Autodesk Inventor part; units mm, degrees
ref_plane "YZ Plane" through (0, 0, 0) normal (1, 0, 0) x (0, 1, 0)
ref_plane "XZ Plane" through (0, 0, 0) normal (0, 1, 0) x (-1, 0, 0)
ref_plane "XY Plane" through (0, 0, 0) normal (0, 0, 1) x (1, 0, 0)
sketch "草圖1" plane through (0, 0, 0) normal (1, 0, 0) x (0, 1, 0)
  line L0 (75, 0) -> (-75, 0)
  line L1 (-75, 0) -> (-75, -300)
  line L2 (-75, -300) -> (75, -300)
  line L3 (75, -300) -> (75, 0)
  circle A0 centre (0, -100) radius 15
  circle A1 centre (0, -150) radius 15
  circle A2 centre (0, -225) radius 30
  line L4 (75, -300) -> (-75, -300)
  line L5 (-75, -300) -> (-75, -725)
  line L6 (-75, -725) -> (75, -725)
  line L7 (75, -725) -> (75, -300)
  point P0 (0, 0)
  point P1 (0, 0)
  dimension "d0" = 150
  dimension "d1" = 300
  dimension "d2" = 200
  dimension "d3" = 50
  dimension "d4" = 75
  dimension "d5" = 60
  dimension "d6" = 30
  dimension "d7" = 500
extrude "擠出1" add sketch "草圖1" along normal mid plane 75
full round fillet "圓角1" first side at (-12.5, -75, -241.6667) centre faces at (12.5, -25, -725) second side at (-12.5, 75, -483.3333)
sketch "草圖2" plane through (37.5, 0, 0) normal (1, 0, 0) x (0, 0, -1)
  arc A0 (650, -75) -> (650, 75) centre (650, 0) ccw
  line L0 (650, 75) -> (0, 75)
  line L1 (0, 75) -> (0, -75)
  line L2 (0, -75) -> (650, -75)
  circle A1 centre (225, 0) radius 30
  circle A2 centre (150, 0) radius 15
  circle A3 centre (100, 0) radius 15
  circle A4 centre (650, 0) radius 200
  point P0 (0, 0)
  dimension "d10" = 400
extrude "擠出2" add sketch "草圖2" along normal blind 30 contours L2 A4 L0 A0 | A0 L0 A4 L2
fillet "圓角2" radius 75 2 edges at (0, 75, 0) (0, -75, 0)
properties part number "震動臂"
Input: part model. Units: mm. Frame: model coordinates. A direction names the side the tool comes from. Coordinates: 2 decimals unless noted, no trailing zeros. Loops run counter-clockwise (first coordinate to the right, second up) from the corner with the lowest first, then second, coordinate; pieces in that order, holes last.
Q1. Material intervals for line 1 (Z direction, x = 4, y = 0); line 2 (X direction, y = 150.5, z = -671.5); line 3 (Y direction, x = 21.5, z = -365.5), sorted ascending.
Q2. Cut plane D-D (y = -153). Output: boundary loops of the cut face in (x, z), then the cut area to 3 significant figures.
Q3. Draft query along Z for faces 5 (the face through (-0.52, 53.61, -702.45)), 6 (the face through (52.29, -8.794, -450.193)), 7 (the face through (-0.525, -3.252, -85.357)). Return one class per face: +Z half, -Z half, draft (parallel to the pull), parting line (faces both ways), or undercut.
Q4. Set-up query: faces 1 (the face through (37.5, 3, -740)), 2 (the face through (-1, -75, -358)), 3 (the face through (-1, 75, -367)), 4 (the face through (-0.52, -52.45, -703.61)). Return all of +Z, -Z, +X, -X, +Y, -Y with unobstructed straight access to the full face (end or side cutting, diameter ignored); none if empty.
Q5. Contact query for flat-ended pins moving along their axis: pin 1 (8 mm diameter, centred on x = 18.5, y = -43, fed in from +Z); pin 2 (4 mm diameter, centred on x = 31, z = -294, fed in from +Y); pin 3 (3 mm diameter, centred on x = 48.5, y = 150, fed in from -Z); pin 4 (24 mm diameter, centred on y = 0, z = -150, fed in from +X). Output: stop coordinate, or through.
Q6. Cut plane B-B (x = -15.5). Give the number of separate pieces and of enclosed holes in the cut face, then the cut area to 3 significant figures.
Q7. Cut plane A-A (z = -225). Output: boundary loops of the cut face in (x, y), then the cut area to 3 significant figures.
Q8. Cut plane C-C (x = 48). Output: boundary loops of the cut face in (y, z), then the cut area to 3 significant figures.
Working result:
1. line 1: z = -725 to -255, -195 to -165, -135 to -115, -85 to 0
1. line 2: x = 37.5 to 67.5
1. line 3: y = -75 to 75
2. outline: (37.5, -778.81) - (67.5, -778.81) - (67.5, -521.19) - (37.5, -521.19) - close
2. area: 7,730 mm2
3. face 5: -Z half
3. face 6: parting line
3. face 7: undercut
4. face 1: -Z, -X
4. face 2: +Z, -Z, -X, -Y
4. face 3: +Z, -Z, -X, +Y
4. face 4: -Z, -X, -Y
5. pin 1: stops at z = -10.94
5. pin 2: stops at y = 75
5. pin 3: stops at z = -783.97
5. pin 4: passes through
6. separate pieces: 1
6. enclosed holes: 3
6. area: 99,700 mm2
7. outline: (-37.5, -75) - (37.5, -75) - (37.5, -30) - (-37.5, -30) - close; (-37.5, 30) - (37.5, 30) - (37.5, 75) - (-37.5, 75) - close
7. area: 6,750 mm2
8. outline: circle Ø400 at (0, -650)
8. area: 126,000 mm2
